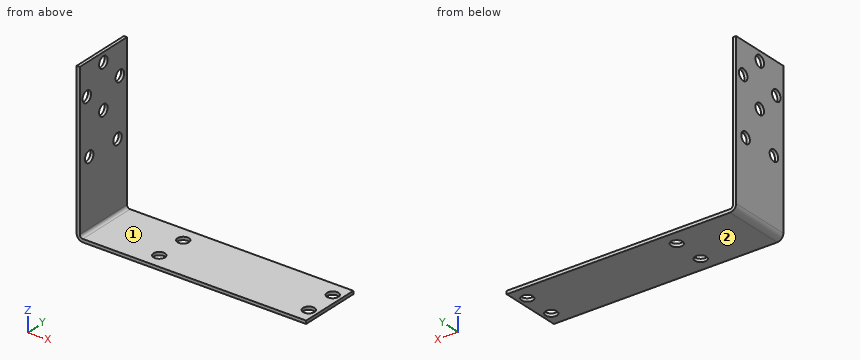
from build123d import *

# Parameters (mm, degrees)
EXTRUDE_1_DEPTH       = 20
SKETCH_22_R           = 1.8
CUT_EXTRUDE_1_DEPTH   = 93.070625066
SKETCH_23_R           = 1.85
CUT_EXTRUDE_2_DEPTH   = 93.876261768
SHEET_METAL_1_DEPTH   = 20
SHEET_METAL_1_2_DEPTH = 20
SKETCH_24_R           = 1.8
CUT_EXTRUDE_3_DEPTH   = 92.268833673


# Read off the part's stored shape, not the designer's step: 转换实体1
with BuildPart() as part:
    # Sketch 1 → 凸台-拉伸1 (new body)
    with BuildSketch(Plane(origin=(0, 0, 0), x_dir=(1, 0, 0), z_dir=(0, 1, 0))):
        Polygon((2, 0), (2, 50), (74, 50), (75, 50), (75, 51), (1, 51), (1, 0), align=None)
    extrude(amount=EXTRUDE_1_DEPTH)

    # 草图22 → 切除-拉伸1 (cut, through all)
    with BuildSketch(Plane.ZY.offset(-1)):
        with Locations((-17, 10)):
            Circle(SKETCH_22_R)
        with Locations((-10, 17)):
            Circle(SKETCH_22_R)
        with Locations((-3, 10)):
            Circle(SKETCH_22_R)
        with Locations((-10, 3)):
            Circle(SKETCH_22_R)
    extrude(amount=-CUT_EXTRUDE_1_DEPTH, mode=Mode.SUBTRACT)

    # 草图23 → 切除-拉伸2 (cut, through all)
    with BuildSketch(Plane(origin=(0, 0, -51), x_dir=(-1, 0, 0), z_dir=(0, 0, -1))):
        with Locations((-72.1, 15.075)):
            Circle(SKETCH_23_R)
        with Locations((-72.1, 4.925)):
            Circle(SKETCH_23_R)
        with Locations((-23.9, 4.925)):
            Circle(SKETCH_23_R)
        with Locations((-23.9, 15.075)):
            Circle(SKETCH_23_R)
    extrude(amount=-CUT_EXTRUDE_2_DEPTH, mode=Mode.SUBTRACT)

    # Sheet Metal 1 outline → Sheet Metal 1 (cut)
    with BuildSketch(Plane(origin=(0, 0, 0), x_dir=(1, 0, 0), z_dir=(0, 1, 0))):
        with BuildLine():
            Line((1, 51), (1, 49))
            ThreePointArc((1, 49), (1.585786438, 50.414213562), (3, 51))
            Line((3, 51), (1, 51))
        make_face()
    extrude(amount=SHEET_METAL_1_DEPTH, mode=Mode.SUBTRACT)

    # Sheet Metal 1 2 outline → Sheet Metal 1 2 (add)
    with BuildSketch(Plane(origin=(0, 0, 0), x_dir=(1, 0, 0), z_dir=(0, 1, 0))):
        with BuildLine():
            Line((2, 50), (2, 49))
            ThreePointArc((2, 49), (2.292893219, 49.707106781), (3, 50))
            Line((3, 50), (2, 50))
        make_face()
    extrude(amount=SHEET_METAL_1_2_DEPTH)

    # 草图24 → 切除-拉伸3 (cut, through all)
    with BuildSketch(Plane(origin=(2, 0, 0), x_dir=(0, 0, -1), z_dir=(1, 0, 0))):
        with Locations((28, 16)):
            Circle(SKETCH_24_R)
        with Locations((28, 4)):
            Circle(SKETCH_24_R)
    extrude(amount=-CUT_EXTRUDE_3_DEPTH, mode=Mode.SUBTRACT)


solid = part.part
Could you check a few things on this model? Use its own coordinates, in mm. Face numbers are marked on the shaded views. A direction names the side the tool comes from. Give positions to 0.01 mm unless a question says otherwise; leave off trailing zeros. Order: outer loops, then holes, each group sorted by start corner. A loop starts at its lowest first (then second) coordinate and runs counter-clockwise, first axis right, second up.
Item 1: I'm going to push flat-ended pins straight in: pin 1 (2 mm diameter, centred on y = 10, z = -17, fed in from +X); pin 2 (5 mm diameter, centred on x = 24, y = 15.5, fed in from +Z); pin 3 (6 mm diameter, centred on y = 3, z = -10, fed in from +X). Where does each tip first touch, or does it pass through?
Item 2: I need wall thicknesses on line 1 (Y direction, x = 1.3, z = -28); line 2 (Y direction, x = 23.9, z = -50.5) (3 decimals); line 3 (Z direction, x = 37, y = 17.75). Which ranges of each line are inside material? Lowest first, please.
Item 3: If we section it at C-C, the plane z = -28: Write out the boundary of the cut face in (x, y), plus the area to 3 significant figures.
Item 4: If we section it at D-D, the plane z = -17: Write out the boundary of the cut face in (x, y).
Item 5: For the marked faces 1 and 2, which set-ups out of +Z, -Z, +X, -X, +Y, -Y let a thin tool reach every point of the face, with its end or its side?
Item 6: If we section it at A-A, the plane x = 23.9: Write out the boundary of the cut face in (y, z) (3 decimals), plus the area to 3 significant figures.
Item 7: If we section it at B-B, the plane y = 10: Write out the boundary of the cut face in (x, z), plus the area to 3 significant figures.
Values:
1. pin 1: passes through
1. pin 2: stops at z = -50
1. pin 3: stops at x = 2
2. line 1: y = 0 to 2.2, 5.8 to 14.2, 17.8 to 20
2. line 2: y = 0 to 3.075, 6.775 to 13.225, 16.925 to 20
2. line 3: z = -51 to -50
3. outline: (1, 0) - (2, 0) - (2, 2.2) - (1, 2.2) - close; (1, 5.8) - (2, 5.8) - (2, 14.2) - (1, 14.2) - close; (1, 17.8) - (2, 17.8) - (2, 20) - (1, 20) - close
3. area: 12.8 mm2
4. outline: (1, 0) - (2, 0) - (2, 8.2) - (1, 8.2) - close; (1, 11.8) - (2, 11.8) - (2, 20) - (1, 20) - close
5. face 1: +Z, +X, +Y, -Y
5. face 2: -Z, +X, -X, +Y, -Y
6. outline: (0, -51) - (3.075, -51) - (3.075, -50) - (0, -50) - close; (6.775, -51) - (13.225, -51) - (13.225, -50) - (6.775, -50) - close; (16.925, -51) - (20, -51) - (20, -50) - (16.925, -50) - close
6. area: 12.6 mm2
7. outline: (1, -49) arc R2 ccw to (3, -51) - (75, -51) - (75, -50) - (3, -50) arc R1 cw to (2, -49) - (2, -18.8) - (1, -18.8) - close; (1, -15.2) - (2, -15.2) - (2, -4.8) - (1, -4.8) - close; (1, -1.2) - (2, -1.2) - (2, 0) - (1, 0) - close
7. area: 116 mm2
